The listing builds one solid part. Answer for the finished solid, in the listing's coordinates (mm). A direction names the side the tool comes from. Coordinates: 2 decimals unless noted, no trailing zeros. Loops run counter-clockwise (first coordinate to the right, second up) from the corner with the lowest first, then second, coordinate; pieces in that order, holes last. Notation, with made-up numbers: M 20,17 L 74,17 A9 ccw 74,34 Z; hole C -3.5,-22.75 d10. An arc over 180 degrees is marked long. Answer as a JSON object with one key per item and string values. Group by question number.
1. A cutting plane is placed at B-B on y = 22. Give the vertices of the cut face in (x, z).
2. Determine the mould class of faces 1 (the face through (-79.912, 36.283, 3.042)), 2 (the face through (20.452, -20.325, 2.958)), 3 (the face through (-27.724, 41, 3)) for opening direction X: released by +X, released by -X, zero draft, split by the parting line, or undercut.
3. Given pin 1 (5 mm diameter, centred on x = 16, y = -5, fed in from -Z); pin 2 (1.5 mm diameter, centred on x = -17, z = 5, fed in from +Y); pin 3 (1 mm diameter, centred on y = 6.5, z = 5, fed in from +X); pin 4 (1.8 mm diameter, centred on x = -31, z = 2.5, fed in from -Y), each flat-ended and moving along its own axis, determine where each tip first touches the part or whether it passes through.
4. A cutting plane is placed at C-C on x = 3. Give the vertices of the cut face in (y, z).
5. A cutting plane is placed at A-A on z = 3.25. Give the vertices of the cut face in (x, y), and give its area (3 significant figures).
6. Straight lines are drawn through the part: L1, parallel to X at y = 12, z = 2.5; L2, parallel to X at y = 15, z = 0.75; L3, parallel to Y at x = 7, z = 4. For each, find the intervals that lie inside material, in ascending order.
7. For faces 4 (the face through (-31, 38.217, 3)), 5 (the face through (-27.724, -29, 3)), 6 (the face through (75.76, 23.31, 2.96)), determine the directions among +Z, -Z, +X, -X, +Y, -Y from which every point of the face is accessible in a straight line to the end or side of a thin tool.
from build123d import *

# Parameters (mm, degrees)
F0_W     = 3
F0_H     = 65
F1_DEPTH = 6
F3_COUNT = 2
F3_ANGLE = 180


with BuildPart() as f1:
    # F0 (on Top) → F1 (new body)
    with BuildSketch(Plane.XY):
        with BuildLine():
            Line((-27.724255, -31.782916), (69.996519, -8.541981))
            ThreePointArc((69.996519, -8.541981), (80.927579, -0.835803), (83.526947, 12.283517))
            ThreePointArc((83.526947, 12.283517), (75.611861, 23.435124), (63.374858, 29.53944))
            Line((63.374858, 29.53944), (-27.724255, 43.217084))
            Line((-27.724255, 43.217084), (-27.724255, 38.217084))
            Line((-27.724255, 38.217084), (-27.724255, -26.782916))
            Line((-27.724255, -26.782916), (-27.724255, -31.782916))
        make_face()
        with Locations((-29.224255, 5.717084)):
            Rectangle(F0_W, F0_H)
    extrude(amount=F1_DEPTH)

    # F3: F1 ×2 about axis
    f3_axis = Axis((-30.724255, 5.717084, 3), (0, -1, 0))


with BuildPart() as f1_1:
    add(f1.part)
    for i in range(1, F3_COUNT):
        add(f1.part.rotate(f3_axis, i * F3_ANGLE / (F3_COUNT - 1)))


solid = f1_1.part
From the geometry:
{
 "1": {"outline": "M -138.61,0 L 77.17,0 L 77.17,6 L -138.61,6 Z"},
 "2": {"face 1": "released by -X", "face 2": "released by +X", "face 3": "undercut"},
 "3": {"pin 1": "stops at z = 0", "pin 2": "stops at y = 41.72", "pin 3": "stops at x = 83.73", "pin 4": "stops at y = -26.78"},
 "4": {"outline": "M -24.48,0 L 38.6,0 L 38.6,6 L -24.48,6 Z"},
 "5": {"outline": "M -144.98,12.28 A18 ccw -131.45,-8.54 L -33.72,-31.78 L -33.72,-26.78 L -27.72,-26.78 L -27.72,-31.78 L 70,-8.54 A18 ccw 83.53,12.28 A28.14 ccw 63.37,29.54 L -27.72,43.22 L -27.72,38.22 L -33.72,38.22 L -33.72,43.22 L -124.82,29.54 A28.14 ccw Z", "area": "12,000 mm²"},
 "6": {"L1": "x = -145.03 to 83.58", "L2": "x = -143.75 to 82.3", "L3": "y = -23.52 to 38"},
 "7": {"face 4": "+Z, -Z, +Y", "face 5": "+Z, -Z, -Y", "face 6": "+Z, -Z, +X, +Y"}
}
